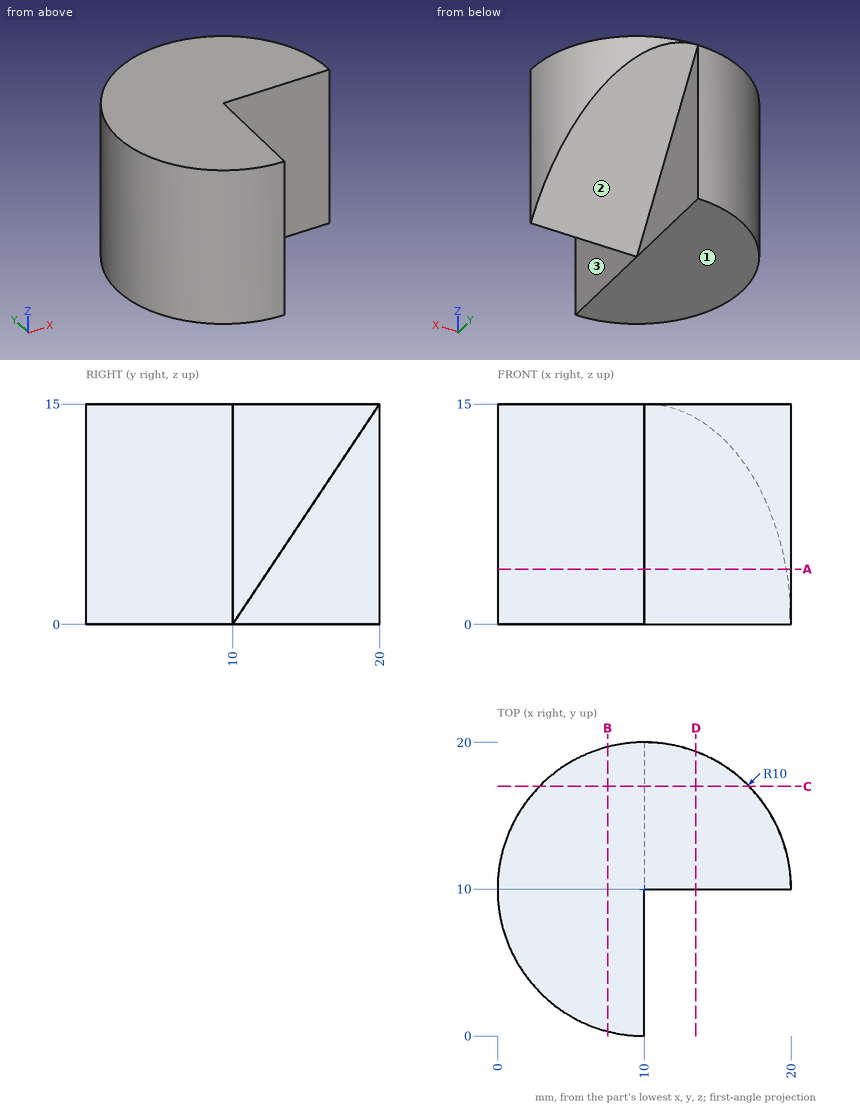
Study the drawing (mm; zero at the part's minimum x, y, z) and answer. A direction names the side the tool comes from. Round coordinates to 2 decimals unless told otherwise and drop trailing zeros. Loops run counter-clockwise (first coordinate to the right, second up) from the corner with the lowest first, then second, coordinate; pieces in that order, holes last. Notation, with made-up numbers: (-35.5, 78.25) -> (19.5, 78.25) arc R21 cw to (19.5, 109.25) -> close; hole circle Ø8 at (-17.75, 19.5). An arc over 180 degrees is marked (long way). Write each question's results on one line, items separated by ' | '. Start each with the question number.
1. Section A-A (z = 3.75) is taken. Determine the outline of the cut face in (x, y).
2. A tool of negligible diameter and unlimited length cuts with its end or side. For the marked faces 1, 2 and 3, from which of +Z, -Z, +X, -X, +Y, -Y can it reach the whole face along a straight path? Write none if from no direction.
3. Section D-D (x = 13.5) is taken. Determine the outline of the cut face in (y, z), plus the area to 3 significant figures.
4. Find the intervals of material crossed by probe 1 along Y at (x, z) = (1.25, 9.5); probe 2 along Y at (x, z) = (17.5, 7.25); probe 3 along X at (y, z) = (2, 9), in increasing order. Write a range as from..to.
5. Given pin 1 Ø1 at (x, z) = (7.5, 10.5) entering from -Y; pin 2 Ø5 at (y, z) = (6.5, 9) entering from +X; pin 3 Ø3 at (x, z) = (2.5, 5) entering from +Y, each flat-ended and moving along its own axis, determine where each tip first touches the part or whether it passes through.
6. Section C-C (y = 17) is taken. Determine the outline of the cut face in (x, z).
7. Section B-B (x = 7.5) is taken. Determine the outline of the cut face in (y, z).
Evaluation:
1) outline: (10, 0) -> (10, 10) -> (20, 10) arc R10 ccw to (19.68, 12.5) -> (10, 12.5) -> (10, 20) arc R10 ccw to start
2) face 1: -Z, +X, -X, +Y, -Y | face 2: -Z, +X, +Y | face 3: +Z, -Z, +X, -Y
3) outline: (10, 0) -> (19.37, 14.05) -> (19.37, 15) -> (10, 15) -> close | area: 74.7 mm2
4) probe 1: y = 5.16..14.84 | probe 2: y = 10..14.83 | probe 3: x = 4..10
5) pin 1: stops at y = 0.2 | pin 2: stops at x = 10 | pin 3: stops at y = 18
6) outline: (2.86, 0) -> (10, 0) -> (10, 10.5) -> (17.14, 10.5) -> (17.14, 15) -> (2.86, 15) -> close
7) outline: (0.32, 0) -> (19.68, 0) -> (19.68, 15) -> (0.32, 15) -> close
